```python
from build123d import *

# Parameters (mm, degrees)
F0_W     = 38.1
F0_H     = 76.2
F1_DEPTH = 277.8125
F2_T     = -2.778125
F3_R     = 3.175
F4_DEPTH = 555.626
F5_W     = 11.1125
F5_H     = 88.9
F6_DEPTH = 76.201


with BuildPart() as f1:
    # F0 (on Top) → F1 (new body, symmetric)
    with BuildSketch(Plane.XY):
        with Locations((19.05, 38.1)):
            Rectangle(F0_W, F0_H)
    extrude(amount=F1_DEPTH, both=True)

    # F2
    f2_openings = [f1.faces().sort_by_distance(p)[0] for p in [
        (38.1, 38.1, 0),
    ]]
    offset(amount=F2_T, openings=f2_openings)

    # F3 (on face) → F4 (cut, through all)
    with BuildSketch(Plane(origin=(0, 0, -277.8125), x_dir=(1, 0, 0), z_dir=(0, 0, -1))):
        with Locations((19.05, -12.7)):
            Circle(F3_R)
        with Locations((19.05, -63.5)):
            Circle(F3_R)
    extrude(amount=-F4_DEPTH, mode=Mode.SUBTRACT)

    # F5 (on face) → F6 (cut, through all)
    with BuildSketch(Plane.XZ):
        with Locations((19.05, -180.975)):
            Rectangle(F5_W, F5_H)
        with Locations((19.05, -60.325)):
            Rectangle(F5_W, F5_H)
        with Locations((19.05, 60.325)):
            Rectangle(F5_W, F5_H)
        with Locations((19.05, 180.975)):
            Rectangle(F5_W, F5_H)
    extrude(amount=-F6_DEPTH, mode=Mode.SUBTRACT)


solid = f1.part
```
Model file for the job. Use its own axes, mm. A direction names the side the tool comes from. Coordinates: 2 decimals unless noted, no trailing zeros. Write each loop counter-clockwise with the first axis right and the second up, starting at its lowest first coordinate (ties: lowest second). Pieces come first, ordered by that corner, then holes. Notation, with made-up numbers: (-26.5, 39) - (10.5, 39) arc R13 cw to (10.5, 47) - close; hole circle Ø1 at (52.5, -28.5). An arc over 180 degrees is marked (long way). One line per item, written item: value. Start each with the question number.
1. Slice it at B-B (x = 8). Write the cut outline in (y, z), plus the area to 3 significant figures.
2. Flat gauge pin, fed straight in: pin 1 (3 mm diameter, centred on y = 40, z = -33, fed in from +X). Where does the tip first touch, or does it go through?
3. Slice it at C-C (y = 35). Write the cut outline in (x, z), plus the area to 3 significant figures.
4. Tool access for faces 1 (the flat face through (20, 39, -275.034)), 2 (the flat face through (19, 0, 4)): list every direction of +Z, -Z, +X, -X, +Y, -Y with a clear straight run to the whole face (end or side of a thin tool).
5. Probe line 1 (Y direction, x = 19, z = -277); line 2 (Z direction, x = 30.5, y = 55.5); line 3 (X direction, y = 12.7, z = 276.35) (3 decimals). List the from-to ranges inside material, lowest first. Write a range as from..to.
6. Mould opens along Z. For faces 3 (the flat face through (0, 38, 4)), 4 (the flat face through (20, 39, 275.034)), 5 (the flat face through (19, 39, 277.812)) say: released by +Z, released by -Z, zero draft, split by the parting line, or undercut.
7. Slice it at A-A (z = -33.5). Write the cut outline in (x, y).
Answers below:
1. outline: (0, -277.81) - (76.2, -277.81) - (76.2, 277.81) - (0, 277.81) - close; hole (2.78, -275.03) - (73.42, -275.03) - (73.42, 275.03) - (2.78, 275.03) - close
1. area: 3,480 mm^2
2. pin 1: stops at x = 2.78
3. outline: (0, -277.81) - (38.1, -277.81) - (38.1, -275.03) - (2.78, -275.03) - (2.78, 275.03) - (38.1, 275.03) - (38.1, 277.81) - (0, 277.81) - close
3. area: 1,740 mm^2
4. face 1: +X
4. face 2: +Z, -Z, +X, -X, -Y
5. line 1: y = 0..9.53, 15.87..60.33, 66.67..76.2
5. line 2: z = -277.81..-275.03, 275.03..277.81
5. line 3: x = 0..15.875, 22.225..38.1
6. face 3: zero draft
6. face 4: undercut
6. face 5: released by +Z
7. outline: (0, 0) - (13.49, 0) - (13.49, 2.78) - (2.78, 2.78) - (2.78, 73.42) - (13.49, 73.42) - (13.49, 76.2) - (0, 76.2) - close; (24.61, 0) - (38.1, 0) - (38.1, 2.78) - (24.61, 2.78) - close; (24.61, 73.42) - (38.1, 73.42) - (38.1, 76.2) - (24.61, 76.2) - close
